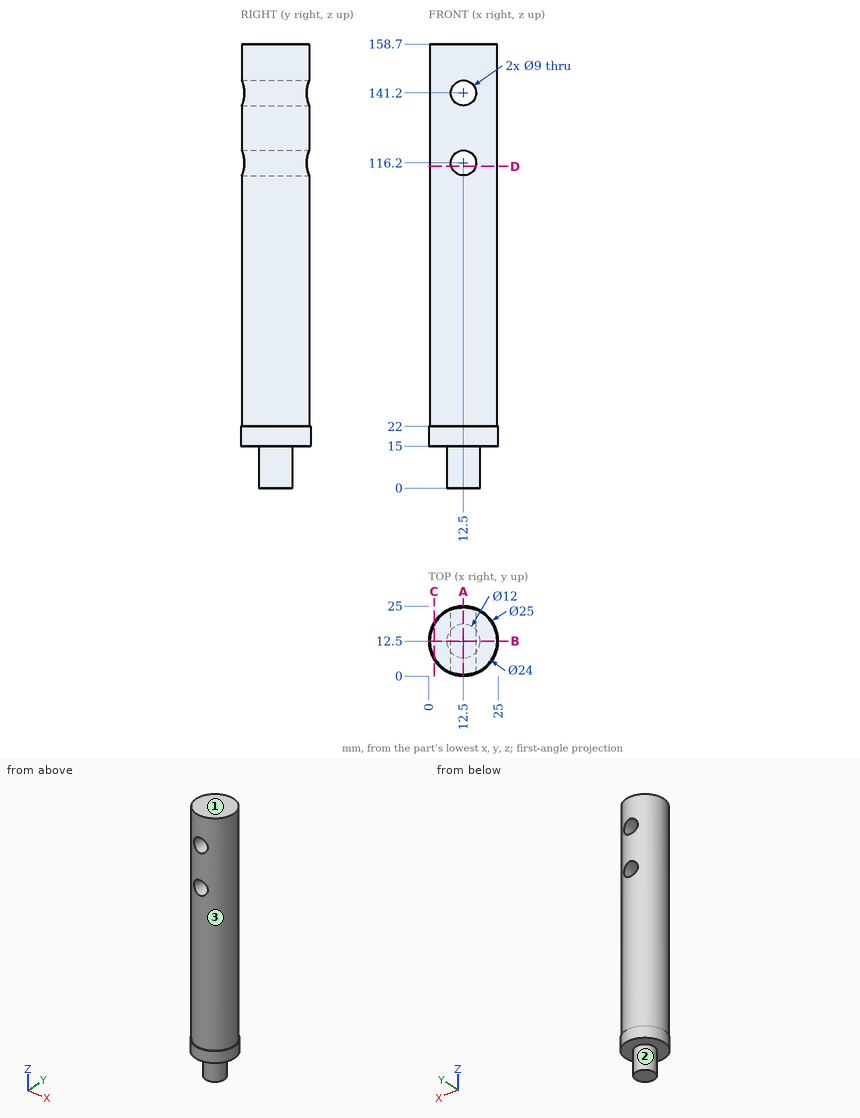
Geometry: see drawing. Coordinates: mm, zero at the bounding-box minimum. A direction names the side the tool comes from. Give positions to 0.01 mm unless a question says otherwise; leave off trailing zeros. Loops run counter-clockwise (first coordinate to the right, second up) from the corner with the lowest first, then second, coordinate; pieces in that order, holes last. Notation, with made-up numbers: (55, -3) - (80, -3) arc R23 cw to (80, 13) - close; hole circle Ø8 at (44.5, -38). An arc over 180 degrees is marked (long way). Use CSV: the item, a comma, the result in double quotes. Start each with the question number.
Item 1: Line query: line 1 (Z direction, x = 12.5, y = 16); line 2 (Z direction, x = 12.5, y = 5.75); line 3 (X direction, y = 12, z = 116.2). Output: solid intervals per line, ascending.
Item 2: Contact query for flat-ended pins moving along their axis: P1, Ø2, axis at y = 16.5, z = 52.5, coming from the -X side; P2, Ø1, axis at y = 11.5, z = 110.5, coming from the -X side; P3, Ø3, axis at x = 14.5, z = 47, coming from the +Y side; P4, Ø5.5, axis at x = 12.5, z = 141.2, coming from the -Y side. Output: stop coordinate, or through.
Item 3: Section C-C on x = 2. Return loops of the section in (y, z).
Item 4: Reachability of the marked faces 1, 2 and 3 from +Z, -Z, +X, -X, +Y, -Y: full face, straight path, thin tool, end or side. Return the list, or none.
Item 5: Section A-A on x = 12.5. Return loops of the section in (y, z), then the cut area to 3 significant figures.
Item 6: Section B-B on y = 12.5. Return loops of the section in (x, z), then the cut area to 3 significant figures.
Item 7: Section D-D on z = 115. Return loops of the section in (x, y), then the cut area to 3 significant figures.
Ans:
1,line 1,"z = 0 to 111.7, 120.7 to 136.7, 145.7 to 158.7"
1,line 2,"z = 15 to 111.7, 120.7 to 136.7, 145.7 to 158.7"
1,line 3,"x = 0.51 to 8, 17 to 24.49"
2,P1,"stops at x = 0.88"
2,P2,"stops at x = 0.51"
2,P3,"stops at y = 24.49"
2,P4,"passes through"
3,outline,"(5.72, 15) - (19.28, 15) - (19.28, 22) - (18.31, 22) - (18.31, 158.7) - (6.69, 158.7) - (6.69, 22) - (5.72, 22) - close"
4,face 1,"+Z, +X, -X, +Y, -Y"
4,face 2,"-Z"
4,face 3,"+Z"
5,outline,"(0, 15) - (6.5, 15) - (6.5, 0) - (18.5, 0) - (18.5, 15) - (25, 15) - (25, 22) - (24.5, 22) - (24.5, 111.7) - (0.5, 111.7) - (0.5, 22) - (0, 22) - close; (0.5, 120.7) - (24.5, 120.7) - (24.5, 136.7) - (0.5, 136.7) - close; (0.5, 145.7) - (24.5, 145.7) - (24.5, 158.7) - (0.5, 158.7) - close"
5,area,"3,200 mm2"
6,outline,"(0, 15) - (6.5, 15) - (6.5, 0) - (18.5, 0) - (18.5, 15) - (25, 15) - (25, 22) - (24.5, 22) - (24.5, 158.7) - (0.5, 158.7) - (0.5, 22) - (0, 22) - close; hole circle Ø9 at (12.5, 116.2); hole circle Ø9 at (12.5, 141.2)"
6,area,"3,510 mm2"
7,outline,"(8.16, 1.31) - (8.16, 23.69) arc R12 ccw to start; (16.84, 1.31) arc R12 ccw to (16.84, 23.69) - close"
7,area,"249 mm2"
